Verification items for the finished model (mm, model axes). Face numbers are marked on the shaded views. Coordinates: 2 decimals unless noted, no trailing zeros. Order: outer loops, then holes, each group sorted by start corner. A loop starts at its lowest first (then second) coordinate and runs counter-clockwise, first axis right, second up. Notation, with made-up numbers: (-12.75, 84.5) -> (40.25, 84.5) arc R24 ccw to (40.25, 109.5) -> close; hole circle Ø7 at (53.5, -4.5). An arc over 180 degrees is marked (long way). Write item = value, one per line. Start each with the question number.
1. Cross-section at C-C on y = -4. Record the cut outline in (x, z).
2. Cross-section at D-D on z = 20.5. Record the cut outline in (x, y), plus the area to 3 significant figures.
3. Go/stop test with flat-tipped pins: P1, Ø1, axis at x = -8, z = 8.5, coming from the +Y side; P2, Ø3, axis at x = 1, z = 24, coming from the +Y side; P3, Ø3, axis at x = -7.5, y = -8, coming from the +Z side; P4, Ø12, axis at y = -9.5, z = 18, coming from the +X side. Record where each tip stops, or that it passes through.
4. Release check for a two-part mould opening along Y. For the marked faces 1, 2 and 3 record: +Y half, -Y half, draft (parallel to the pull), parting line (faces both ways), or undercut.
5. Thickness scan on line 1 along Y through (x, z) = (0, 25.75); line 2 along Z through (x, y) = (6, -6); line 3 along Y through (x, z) = (0, 1.85). Record the ranges inside material, lowest first. Write a range as from..to.
6. Cross-section at B-B on x = 0. Record the cut outline in (y, z).
7. Cross-section at A-A on y = 0. Record the cut outline in (x, z).
from build123d import *

# Parameters (mm, degrees)
SKETCH_1_R      = 15.6
SKETCH_1_R_2    = 12.6
SKETCH_1_R_3    = 6.3
SKETCH_1_R_4    = 1.65
EXTRUDE_1_DEPTH = 3
SKETCH_2_R      = 15.6
SKETCH_2_R_2    = 12.7
EXTRUDE_2_DEPTH = 30


with BuildPart() as part:
    # 草图1 → 凸台-拉伸1 (new body)
    # profile 1 of 2: a face of its own
    with BuildSketch(Plane.XY):
        Circle(SKETCH_1_R)
        Circle(SKETCH_1_R_2, mode=Mode.SUBTRACT)
    # profile 2 of 2: a face of its own
    with BuildSketch(Plane.XY):
        Circle(SKETCH_1_R_2)
        Circle(SKETCH_1_R_3, mode=Mode.SUBTRACT)
        with Locations((-9, 0)):
            Circle(SKETCH_1_R_4, mode=Mode.SUBTRACT)
        with Locations((9, 0)):
            Circle(SKETCH_1_R_4, mode=Mode.SUBTRACT)
    extrude(amount=EXTRUDE_1_DEPTH)

    # 草图2 → 凸台-拉伸2 (add)
    with BuildSketch(Plane.XY.offset(3)):
        Circle(SKETCH_2_R)
        Circle(SKETCH_2_R_2, mode=Mode.SUBTRACT)
    extrude(amount=EXTRUDE_2_DEPTH)


solid = part.part
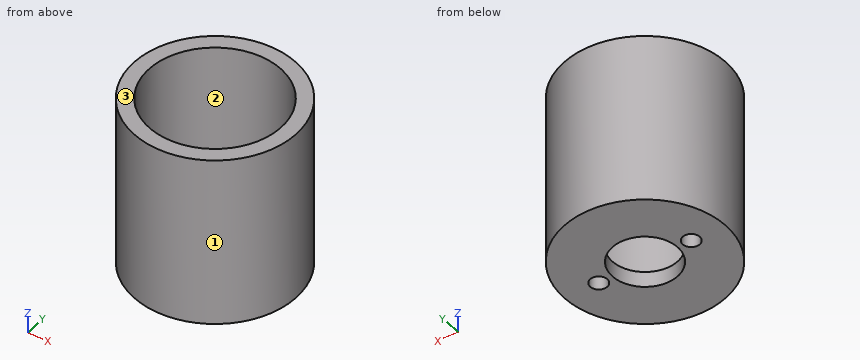
Worked out:
q1.outline = (-15.08, 0) -> (-4.87, 0) -> (-4.87, 3) -> (-12.05, 3) -> (-12.05, 33) -> (-15.08, 33) -> close; (4.87, 0) -> (15.08, 0) -> (15.08, 33) -> (12.05, 33) -> (12.05, 3) -> (4.87, 3) -> close
q2.outline = circle Ø31.2 at (0, 0); hole circle Ø25.4 at (0, 0)
q2.area = 258 mm²
q3.P1 = 13.68
q3.P2 = 15.6
q3.P3 = 3
q3.P4 = 15.2
q4.face_1 = parting line
q4.face_2 = undercut
q4.face_3 = draft
q5.line_1 = -15.6..-12.7, 12.7..15.6
q5.line_2 = 0..3
q5.line_3 = -15.6..-6.3, 6.3..15.6
q6.outline = (-15.6, 0) -> (-6.3, 0) -> (-6.3, 3) -> (-12.7, 3) -> (-12.7, 33) -> (-15.6, 33) -> close; (6.3, 0) -> (15.6, 0) -> (15.6, 33) -> (12.7, 33) -> (12.7, 3) -> (6.3, 3) -> close
q7.outline = (-15.6, 0) -> (-10.65, 0) -> (-10.65, 3) -> (-12.7, 3) -> (-12.7, 33) -> (-15.6, 33) -> close; (-7.35, 0) -> (-6.3, 0) -> (-6.3, 3) -> (-7.35, 3) -> close; (6.3, 0) -> (7.35, 0) -> (7.35, 3) -> (6.3, 3) -> close; (10.65, 0) -> (15.6, 0) -> (15.6, 33) -> (12.7, 33) -> (12.7, 3) -> (10.65, 3) -> close
